```python
from build123d import *

# Parameters (mm, degrees)
F0_R     = 3.65
F1_DEPTH = 44.45
F3_W     = 34.925
F3_H     = 38.1
F4_DEPTH = 22.225
F5_SIZE  = 0.508
F2_R     = 12.7
F2_R_2   = 9.525
F6_DEPTH = 6.35
F7_DEPTH = 25.4
F8_R     = 5.08


with BuildPart() as f1:
    # F0 (on Right) → F1 (new body)
    with BuildSketch(Plane.YZ):
        with BuildLine():
            Line((-17.78, 0), (0, 0))
            Line((0, 0), (0, 68.2625))
            ThreePointArc((0, 68.2625), (-8.89, 77.1525), (-17.78, 68.2625))
            Line((-17.78, 68.2625), (-17.78, 0))
        make_face()
        with Locations((-8.89, 68.2625)):
            Circle(F0_R, mode=Mode.SUBTRACT)
    extrude(amount=F1_DEPTH)

    # F3 (on Front) → F4 (join)
    with BuildSketch(Plane.XZ):
        with Locations((22.225, 31.75)):
            Rectangle(F3_W, F3_H)
    extrude(amount=F4_DEPTH)

    # F5
    f5_edges = [f1.edges().sort_by_distance(p)[0] for p in [
        (4.7625, -22.225, 31.75),
        (22.225, -22.225, 50.8),
        (22.225, -22.225, 12.7),
        (39.6875, -22.225, 31.75),
    ]]
    chamfer(f5_edges, length=F5_SIZE)

    # F2 (on Front) → F6 (cut)
    with BuildSketch(Plane.XZ):
        with Locations((22.225, 31.75)):
            Circle(F2_R)
        with Locations((22.225, 31.75)):
            Circle(F2_R_2, mode=Mode.SUBTRACT)
    extrude(amount=F6_DEPTH, mode=Mode.SUBTRACT)

    # F2 (on Front) → F7 (cut)
    with BuildSketch(Plane.XZ):
        with Locations((22.225, 31.75)):
            Circle(F2_R_2)
    extrude(amount=F7_DEPTH, mode=Mode.SUBTRACT)

    # F8
    f8_edges = [f1.edges().sort_by_distance(p)[0] for p in [
        (0, -8.89, 0),
        (44.45, -8.89, 0),
    ]]
    fillet(f8_edges, radius=F8_R)


solid = f1.part
```
Here's how the part is built. I have some questions about the finished solid (model axes, mm). A direction names the side the tool comes from. Give positions to 0.01 mm unless a question says otherwise; leave off trailing zeros. Use a Markdown table: item, result. Add a question column.
1. Suppose I cut it at A-A (y = -8.89). Give the number of separate pieces and of enclosed holes in the cut face, and give its area (3 significant figures).
2. If we mould it in two halves opening along Z, with no side actions, what happens to faces 4 (the cylindrical face through (1.449, -8.766, 1.528)), 5 (the flat face through (44.45, -9, 42)), 6 (the cylindrical face through (20.16, -14.18, 22.45))? For each: +Z half, -Z half, draft (parallel to the pull), parting line (faces both ways), or undercut.
3. For pin 1 Ø5 at (x, y) = (31.5, -2.5) entering from +Z; pin 2 Ø5 at (x, y) = (30.5, -3) entering from +Z; pin 3 Ø3 at (x, y) = (20, -20.5) entering from +Z, each with a flat end and sliding along its axis, tell me the tip position at first contact or that it passes through.
4. I need wall thicknesses on probe 1 along Z at (x, y) = (12.5, -8.89); probe 2 along Z at (x, y) = (13.5, -8.89); probe 3 along X at (y, z) = (-12, 31.75). Which ranges of each line are inside material? Lowest first, please. Write a range as from..to.
5. On a 3-axis mill with a long thin cutter (end or side, diameter ignored), from which of +Z, -Z, +X, -X, +Y, -Y can I reach the whole of each face in a straight line? I mean faces 1 (the flat face through (39.688, -20, 31)), 2 (the flat face through (22, -20, 50.8)), 3 (the cylindrical face through (19.472, -3.131, 19.352)). Say none if no direction works.
Results list:
| question | item | result |
|---|---|---|
| 1 | separate pieces | 2 |
| 1 | enclosed holes | 1 |
| 1 | area | 2,810 mm² |
| 2 | face 4 | -Z half |
| 2 | face 5 | draft |
| 2 | face 6 | undercut |
| 3 | pin 1 | stops at z = 76.26 |
| 3 | pin 2 | stops at z = 76.48 |
| 3 | pin 3 | stops at z = 50.8 |
| 4 | probe 1 | z = 0..64.61, 71.91..77.15 |
| 4 | probe 2 | z = 0..27.93, 35.57..64.61, 71.91..77.15 |
| 4 | probe 3 | x = 0..12.7, 31.75..44.45 |
| 5 | face 1 | +Z, -Z, +X, -Y |
| 5 | face 2 | +Z, +X, -X, -Y |
| 5 | face 3 | +Y |
